Could you check a few things on this model? Use its own coordinates, in mm. Face numbers are marked on the shaded views. A direction names the side the tool comes from. Coordinates: 2 decimals unless noted, no trailing zeros. Write each loop counter-clockwise with the first axis right and the second up, starting at its lowest first coordinate (ties: lowest second). Pieces come first, ordered by that corner, then holes. Notation, with made-up numbers: M 46,-16.75 L 64,-16.75 A26 ccw 64,11.25 Z; hole C -14,-10.5 d5. An arc over 180 degrees is marked long. Answer as CSV lines item,"result". Start each with the question number.
Item 1: On a 3-axis mill with a long thin cutter (end or side, diameter ignored), from which of +Z, -Z, +X, -X, +Y, -Y can I reach the whole of each face in a straight line? I mean the marked faces 1, 2, 3 and 4. Say none if no direction works.
Item 2: Suppose I cut it at D-D, the plane z = 6.75. State how many separate pieces and enclosed holes the cut face has, and give its area (3 significant figures).
Item 3: We'd pull the mould along Y, two halves only. Please class the marked faces 5, 6 and 7: +Y half, -Y half, draft (parallel to the pull), parting line (faces both ways), or undercut.
Item 4: Suppose I cut it at C-C, the plane y = -21. Write out the boundary of the cut face in (x, z).
Item 5: Suppose I cut it at B-B, the plane z = -1. Write out the boundary of the cut face in (x, y) (3 decimals).
Item 6: Suppose I cut it at A-A, the plane x = -5.5. Write out the boundary of the cut face in (y, z), and give its area (3 significant figures).
Item 7: If I drill on line 1 along Y through (x, z) = (0, 1.35); line 2 along Y through (x, z) = (23, 5.75); line 3 along Z through (x, y) = (24.5, -19.5), over which ranges is the centre line in solid material (lowest first)? Write a range as [from, to].
Item 8: I'm going to push flat-ended pins straight in: P1, Ø4, axis at x = -31.5, y = -31, coming from the -Z side; P2, Ø0.8, axis at y = -2, z = -1.5, coming from the -X side; P3, Ø5.5, axis at x = 0, y = -2, coming from the +Z side; P4, Ø1.4, axis at y = -1.5, z = -2, coming from the +X side. Where does each tip first touch, or does it pass through?
```python
from build123d import *

# Parameters (mm, degrees)
F0_W     = 55
F0_H     = 11
F0_H_2   = 5
F1_DEPTH = 8
F0_R     = 1.75
F2_DEPTH = 4
F3_DEPTH = 3.5
F0_W_2   = 48.086722
F0_H_3   = 22
F4_DEPTH = 8


with BuildPart() as f1:
    # F0 (on Top) → F1 (new body)
    with BuildSketch(Plane.XY):
        with Locations((0, -2.5)):
            Rectangle(F0_W, F0_H)
        Polygon((-22.38157, -0.625), (-20, 0.75), (-17.61843, -0.625), (-17.61843, -3.375), (-20, -4.75), (-22.38157, -3.375), align=None, mode=Mode.SUBTRACT)
        Polygon((-2.38157, -0.625), (0, 0.75), (2.38157, -0.625), (2.38157, -3.375), (0, -4.75), (-2.38157, -3.375), align=None, mode=Mode.SUBTRACT)
        Polygon((17.61843, -0.625), (20, 0.75), (22.38157, -0.625), (22.38157, -3.375), (20, -4.75), (17.61843, -3.375), align=None, mode=Mode.SUBTRACT)
        with Locations((0, 5.5)):
            Rectangle(F0_W, F0_H_2)
    extrude(amount=F1_DEPTH)

    # F0 (on Top) → F2 (join)
    with BuildSketch(Plane.XY):
        Polygon((2.38157, -0.625), (0, 0.75), (-2.38157, -0.625), (-2.38157, -3.375), (0, -4.75), (2.38157, -3.375), align=None)
        with Locations((0, -2)):
            Circle(F0_R, mode=Mode.SUBTRACT)
        Polygon((22.38157, -0.625), (20, 0.75), (17.61843, -0.625), (17.61843, -3.375), (20, -4.75), (22.38157, -3.375), align=None)
        with Locations((20, -2)):
            Circle(F0_R, mode=Mode.SUBTRACT)
        Polygon((-17.61843, -0.625), (-20, 0.75), (-22.38157, -0.625), (-22.38157, -3.375), (-20, -4.75), (-17.61843, -3.375), align=None)
        with Locations((-20, -2)):
            Circle(F0_R, mode=Mode.SUBTRACT)
    extrude(amount=F2_DEPTH)

    # F0 (on Top) → F3 (join)
    with BuildSketch(Plane.XY):
        with Locations((0, -2.5)):
            Rectangle(F0_W, F0_H)
        Polygon((-22.38157, -0.625), (-20, 0.75), (-17.61843, -0.625), (-17.61843, -3.375), (-20, -4.75), (-22.38157, -3.375), align=None, mode=Mode.SUBTRACT)
        Polygon((-2.38157, -0.625), (0, 0.75), (2.38157, -0.625), (2.38157, -3.375), (0, -4.75), (-2.38157, -3.375), align=None, mode=Mode.SUBTRACT)
        Polygon((17.61843, -0.625), (20, 0.75), (22.38157, -0.625), (22.38157, -3.375), (20, -4.75), (17.61843, -3.375), align=None, mode=Mode.SUBTRACT)
    extrude(amount=-F3_DEPTH)

    # F0 (on Top) → F4 (join)
    with BuildSketch(Plane.XY):
        with BuildLine():
            Line((27.5, -8), (-27.5, -8))
            ThreePointArc((-27.5, -8), (-32.483751, -29.904804), (-51.967503, -41.087007))
            Line((-51.967503, -41.087007), (51.967503, -41.087007))
            ThreePointArc((51.967503, -41.087007), (32.483751, -29.904804), (27.5, -8))
        make_face()
        with Locations((0, -25.087007)):
            Rectangle(F0_W_2, F0_H_3, mode=Mode.SUBTRACT)
    extrude(amount=F4_DEPTH)


solid = f1.part
```
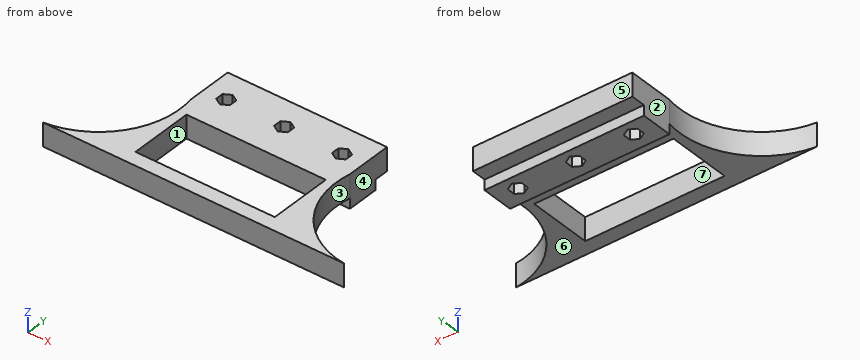
Ans:
1,face 1,"+Z, -Z"
1,face 2,"+Z, -Z, -X, +Y"
1,face 3,"+Z, -Z, +X"
1,face 4,"+Z, -Z, +X, +Y"
2,separate pieces,"1"
2,enclosed holes,"4"
2,area,"1,880 mm^2"
3,face 5,"+Y half"
3,face 6,"draft"
3,face 7,"undercut"
4,outline,"M -28.09,0 L -24.04,0 L -24.04,8 L -28.09,8 Z; M 24.04,0 L 28.09,0 L 28.09,8 L 24.04,8 Z"
5,outline,"M -27.5,-8 L 27.5,-8 L 27.5,3 L -27.5,3 Z; hole M -22.382,-3.375 L -20,-4.75 L -17.618,-3.375 L -17.618,-0.625 L -20,0.75 L -22.382,-0.625 Z; hole M -2.382,-3.375 L 0,-4.75 L 2.382,-3.375 L 2.382,-0.625 L 0,0.75 L -2.382,-0.625 Z; hole M 17.618,-3.375 L 20,-4.75 L 22.382,-3.375 L 22.382,-0.625 L 20,0.75 L 17.618,-0.625 Z"
6,outline,"M -41.09,0 L -36.09,0 L -36.09,8 L -41.09,8 Z; M -14.09,0 L -8,0 L -8,-3.5 L 3,-3.5 L 3,0 L 8,0 L 8,8 L -14.09,8 Z"
6,area,"255 mm^2"
7,line 1,"y = [-41.09, -36.09], [-14.09, -3.75], [-0.25, 8]"
7,line 2,"y = [-41.09, -36.09], [-14.09, 8]"
7,line 3,"z = [0, 8]"
8,P1,"stops at z = 0"
8,P2,"stops at x = -27.5"
8,P3,"stops at z = 8"
8,P4,"stops at x = 27.5"
